Geometry check sheet. Reference: drawing and pictorial views, mm from the part's lowest x, y, z. A direction names the side the tool comes from. Give positions to 0.01 mm unless a question says otherwise; leave off trailing zeros. Order: outer loops, then holes, each group sorted by start corner. A loop starts at its lowest first (then second) coordinate and runs counter-clockwise, first axis right, second up.
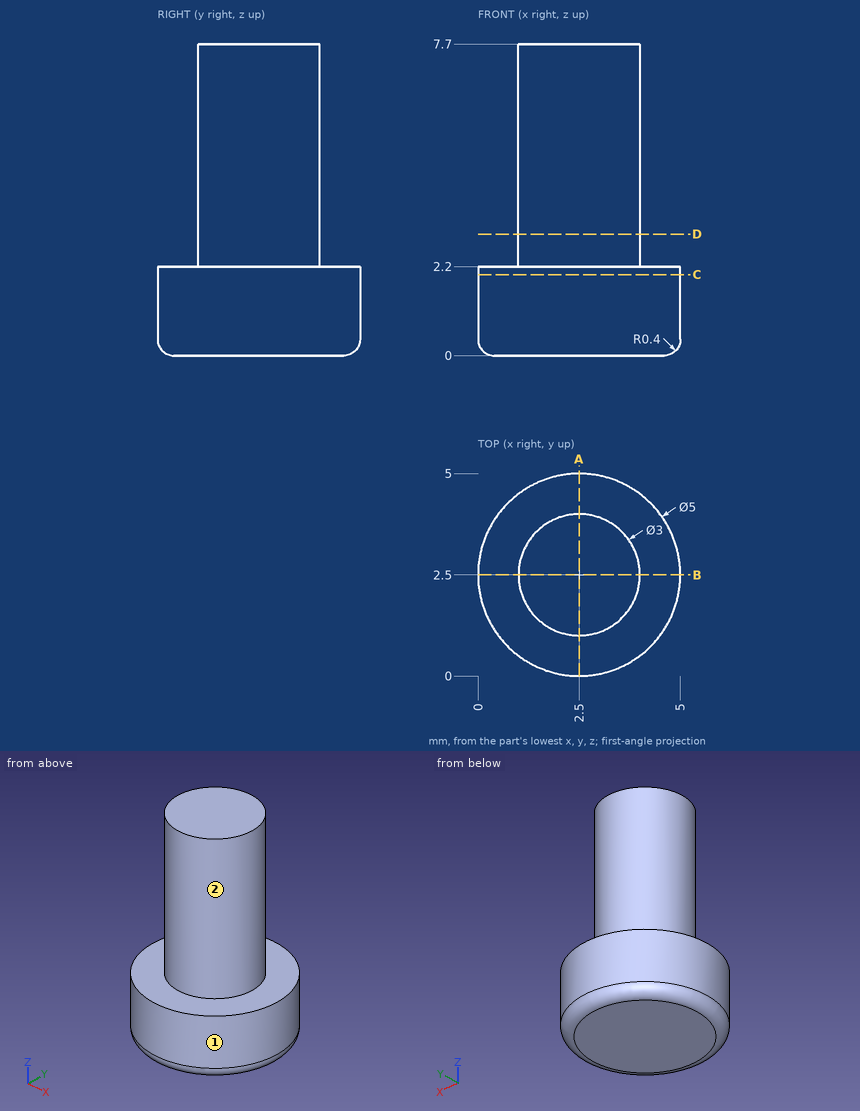
1) Material ranges on L1, parallel to Z at x = 3.9, y = 4.1; L2, parallel to X at y = 4.5, z = 1; L3, parallel to X at y = 1.3, z = 2, recorded low to high.
Recorded:
L1: z = 0 to 2.2
L2: x = 1 to 4
L3: x = 0.31 to 4.69
2) Section check A-A, the plane x = 2.5. Record the cut outline in (y, z).
Recorded:
outline: (0, 0.4) arc R0.4 ccw to (0.4, 0) - (4.6, 0) arc R0.4 ccw to (5, 0.4) - (5, 2.2) - (4, 2.2) - (4, 7.7) - (1, 7.7) - (1, 2.2) - (0, 2.2) - close
3) Set-up check for the marked faces 1 and 2: record each of +Z, -Z, +X, -X, +Y, -Y from which the full face is reachable in a straight line by a thin tool's end or side.
Recorded:
face 1: +Z, -Z
face 2: +Z
4) Section check C-C, the plane z = 2. Record the cut outline in (x, y), then the cut area to 3 significant figures.
Recorded:
outline: circle Ø5 at (2.5, 2.5)
area: 19.6 mm2
5) Depth check by flat-ended pin: pin 1 Ø2 at (y, z) = (0.5, 6.5) entering from -X; pin 2 Ø1 at (x, z) = (1.5, 1.5) entering from -Y. Enter the tip coordinate at first touch or a pass-through.
Recorded:
pin 1: stops at x = 1.38
pin 2: stops at y = 0.05
6) Section check D-D, the plane z = 3. Record the cut outline in (x, y).
Recorded:
outline: circle Ø3 at (2.5, 2.5)
